from build123d import *


with BuildPart() as f1:
    # F0 (on Front) → F1 (revolve)
    with BuildSketch(Plane.XZ):
        Polygon((0, 17.5), (0, 0), (133.846119, 0), (133.846119, 17.5), (93.846119, 17.5), (93.846119, 30), (73.846136, 30), (73.846136, 17.5), align=None)
    revolve(axis=Axis((66.923059, 0, 0), (-1, 0, 0)))

    # F2: F1 across face


with BuildPart() as f1_1:
    add(f1.part)
    add(f1.part.mirror(Plane(origin=(0, 0, 0), x_dir=(0, -1, 0), z_dir=(-1, 0, 0))))


solid = f1_1.part
Verification items for the finished model (mm, model axes). A direction names the side the tool comes from. Give positions to 0.01 mm unless a question says otherwise; leave off trailing zeros. Loops run counter-clockwise (first coordinate to the right, second up) from the corner with the lowest first, then second, coordinate; pieces in that order, holes last.
1) Draft check along X on faces 1 (the cylindrical face through (-113.566, -10.648, -13.887)), 2 (the flat face through (133.846, 0, 0)), 3 (the flat face through (73.846, -13, 13)). Enter one of: pulls with the +X half, pulls with the -X half, needs draft (parallel to the pull), parting line crosses it, or undercut.
2) Thickness scan on line 1 along X through (y, z) = (9.5, -23); line 2 along Z through (x, y) = (-118, 4.5); line 3 along Y through (x, z) = (11.5, -10). Record the ranges inside material, lowest first.
3) Sectioned sample at D-D, the plane z = -24.5. Enter the section's corners in (x, y).
4) Depth check by flat-ended pin: pin 1 Ø4 at (x, z) = (-88.5, 1.5) entering from +Y; pin 2 Ø1.5 at (x, z) = (-105, -5) entering from +Y; pin 3 Ø1.5 at (x, y) = (-68, 3.5) entering from -Z. Enter the tip coordinate at first touch or a pass-through.
5) Set-up check for faces 4 (the flat face through (-93.846, -13, -13)), 5 (the flat face through (-133.846, 0, 0)), 6 (the flat face through (-73.846, -13, 13)), 7 (the cylindrical face through (-83.71, 1.32, -29.97)), 8 (the cylindrical face through (113.566, -10.648, -13.887)): record each of +Z, -Z, +X, -X, +Y, -Y from which the full face is reachable in a straight line by a thin tool's end or side.
6) Sectioned sample at C-C, the plane y = -22. Enter the section's corners in (x, z), then the cut area to 3 significant figures.
7) Sectioned sample at A-A, the plane z = 0. Enter the section's corners in (x, y).
Answers:
1. face 1: needs draft
1. face 2: pulls with the +X half
1. face 3: undercut
2. line 1: x = -93.85 to -73.85, 73.85 to 93.85
2. line 2: z = -16.91 to 16.91
2. line 3: y = -14.36 to 14.36
3. outline: (-93.85, -17.31) - (-73.85, -17.31) - (-73.85, 17.31) - (-93.85, 17.31) - close; (73.85, -17.31) - (93.85, -17.31) - (93.85, 17.31) - (73.85, 17.31) - close
4. pin 1: stops at y = 30
4. pin 2: stops at y = 16.98
4. pin 3: stops at z = -17.28
5. face 4: -X
5. face 5: +Z, -Z, -X, +Y, -Y
5. face 6: none
5. face 7: +X, -X
5. face 8: +X
6. outline: (-93.85, -20.4) - (-73.85, -20.4) - (-73.85, 20.4) - (-93.85, 20.4) - close; (73.85, -20.4) - (93.85, -20.4) - (93.85, 20.4) - (73.85, 20.4) - close
6. area: 1,630 mm2
7. outline: (-133.85, -17.5) - (-93.85, -17.5) - (-93.85, -30) - (-73.85, -30) - (-73.85, -17.5) - (73.85, -17.5) - (73.85, -30) - (93.85, -30) - (93.85, -17.5) - (133.85, -17.5) - (133.85, 17.5) - (93.85, 17.5) - (93.85, 30) - (73.85, 30) - (73.85, 17.5) - (-73.85, 17.5) - (-73.85, 30) - (-93.85, 30) - (-93.85, 17.5) - (-133.85, 17.5) - close
